```python
from build123d import *

# Parameters (mm, degrees)
SKETCH1_W           = 200
SKETCH1_H           = 200
BOSS_EXTRUDE1_DEPTH = 15
SKETCH2_R           = 70
BOSS_EXTRUDE2_DEPTH = 90
SKETCH4_R           = 65
CUT_EXTRUDE1_DEPTH  = 3
SKETCH5_W           = 85
SKETCH5_H           = 38
BOSS_EXTRUDE3_DEPTH = 100
SKETCH6_R           = 5
CUT_EXTRUDE2_DEPTH  = 15


with BuildPart() as part:
    # Sketch1 → Boss-Extrude1 (new body)
    with BuildSketch(Plane(origin=(0, 0, 0), x_dir=(1, 0, 0), z_dir=(0, 1, 0))):
        Rectangle(SKETCH1_W, SKETCH1_H)
    extrude(amount=BOSS_EXTRUDE1_DEPTH)

    # Sketch2 → Boss-Extrude2 (add)
    with BuildSketch(Plane(origin=(0, 15, 0), x_dir=(1, 0, 0), z_dir=(0, 1, 0))):
        with Locations(Location((0, 0, 0), (0, 0, 90))):
            Circle(SKETCH2_R)
    extrude(amount=BOSS_EXTRUDE2_DEPTH)

    # Sketch4 → Cut-Extrude1 (cut)
    with BuildSketch(Plane(origin=(0, 105, 0), x_dir=(1, 0, 0), z_dir=(0, 1, 0))):
        with Locations(Location((0, 0, 0), (0, 0, 270))):
            Circle(SKETCH4_R)
    extrude(amount=-CUT_EXTRUDE1_DEPTH, mode=Mode.SUBTRACT)

    # Sketch5 → Boss-Extrude3 (add)
    with BuildSketch(Plane(origin=(0, 0, 0), x_dir=(0, 0, -1), z_dir=(1, 0, 0))):
        with Locations((0, 59)):
            Rectangle(SKETCH5_W, SKETCH5_H)
    extrude(amount=BOSS_EXTRUDE3_DEPTH)

    # Sketch6 → Cut-Extrude2 (cut)
    with BuildSketch(Plane.XZ):
        with Locations(Location((-90, 90, 0), (0, 0, 270))):
            Circle(SKETCH6_R)
        with Locations(Location((0, 90, 0), (0, 0, 270))):
            Circle(SKETCH6_R)
        with Locations(Location((90, 90, 0), (0, 0, 270))):
            Circle(SKETCH6_R)
        with Locations(Location((90, 0, 0), (0, 0, 270))):
            Circle(SKETCH6_R)
        with Locations(Location((90, -90, 0), (0, 0, 270))):
            Circle(SKETCH6_R)
        with Locations(Location((-90, -90, 0), (0, 0, 270))):
            Circle(SKETCH6_R)
        with Locations(Location((-90, 0, 0), (0, 0, 270))):
            Circle(SKETCH6_R)
        with Locations(Location((0, -90, 0), (0, 0, 270))):
            Circle(SKETCH6_R)
    extrude(amount=-CUT_EXTRUDE2_DEPTH, mode=Mode.SUBTRACT)


solid = part.part
```
Geometry: final body of the model. Coordinates: model frame, mm. A direction names the side the tool comes from. Coordinates: 2 decimals unless noted, no trailing zeros. Order: outer loops, then holes, each group sorted by start corner. A loop starts at its lowest first (then second) coordinate and runs counter-clockwise, first axis right, second up. Notation, with made-up numbers: (0, 15) - (12, 15) arc R31 cw to (12, 45) - close; hole circle Ø3 at (-36, -17). An arc over 180 degrees is marked (long way). Write each question's results on one line, items separated by ' | '.
(1) Section query C-C, the plane y = 12. Count the separate pieces of the cut face and the enclosed holes in it, plus the area to 3 significant figures.
Values found:
separate pieces: 1 | enclosed holes: 8 | area: 39,400 mm²
(2) Section query B-B, the plane x = 0. Return the cut outline in (y, z), plus the area to 3 significant figures.
Values found:
outline: (0, -100) - (15, -100) - (15, -95) - (0, -95) - close; (0, -85) - (15, -85) - (15, -70) - (105, -70) - (105, -65) - (102, -65) - (102, 65) - (105, 65) - (105, 70) - (15, 70) - (15, 85) - (0, 85) - close; (0, 95) - (15, 95) - (15, 100) - (0, 100) - close | area: 14,900 mm²
(3) First-contact query: pin 1 Ø11.5 at (x, y) = (87.5, 58) entering from -Z; pin 2 Ø13 at (x, z) = (0, 90) entering from +Y; pin 3 Ø6 at (x, z) = (90, 0) entering from +Y. Flat tips, straight axial feed; report the tip coordinate or a pass-through.
Values found:
pin 1: stops at z = -42.5 | pin 2: stops at y = 15 | pin 3: stops at y = 78
(4) Line query: line 1 (X direction, y = 11, z = 90); line 2 (X direction, y = 4.25, z = 0); line 3 (Y direction, x = 82, z = 10). Output: solid intervals per line, ascending. Write a range as [from, to].
Values found:
line 1: x = [-100, -95], [-85, -5], [5, 85], [95, 100] | line 2: x = [-100, -95], [-85, 85], [95, 100] | line 3: y = [0, 15], [40, 78]
(5) Mould query, pull axis X, two halves, no side actions, for faces 1 (the face through (88.085, 7.395, -94.619)), 2 (the face through (100, 7, 1)), 3 (the face through (-1, 7, -100)). Classes: +X half, -X half, draft (parallel to the pull), parting line (faces both ways), or undercut.
Values found:
face 1: undercut | face 2: +X half | face 3: draft
(6) Set-up query: faces 4 (the face through (-100, 7, 1)), 5 (the face through (85.12, 7.4, 1.08)), 6 (the face through (78, 59, 42.5)), 7 (the face through (19.52, 103.52, 62)), 8 (the face through (78, 59, -42.5)). Return all of +Z, -Z, +X, -X, +Y, -Y with unobstructed straight access to the full face (end or side cutting, diameter ignored); none if empty.
Values found:
face 4: +Z, -Z, -X, +Y, -Y | face 5: -Y | face 6: +Z, +X, +Y | face 7: +Y | face 8: -Z, +X, +Y
(7) Section query A-A, the plane z = -90. Return the cut outline in (x, y), plus the area to 3 significant figures.
Values found:
outline: (-100, 0) - (-95, 0) - (-95, 15) - (-100, 15) - close; (-85, 0) - (-5, 0) - (-5, 15) - (-85, 15) - close; (5, 0) - (85, 0) - (85, 15) - (5, 15) - close; (95, 0) - (100, 0) - (100, 15) - (95, 15) - close | area: 2,550 mm²
(8) Section query D-D, the plane z = 0. Return the cut outline in (x, y).
Values found:
outline: (-100, 0) - (-95, 0) - (-95, 15) - (-100, 15) - close; (-85, 0) - (85, 0) - (85, 15) - (70, 15) - (70, 40) - (100, 40) - (100, 78) - (70, 78) - (70, 105) - (65, 105) - (65, 102) - (-65, 102) - (-65, 105) - (-70, 105) - (-70, 15) - (-85, 15) - close; (95, 0) - (100, 0) - (100, 15) - (95, 15) - close
